Autodesk Inventor part; units mm, degrees
ref_plane "YZ Plane" through (0, 0, 0) normal (1, 0, 0) x (0, 1, 0)
ref_plane "XZ Plane" through (0, 0, 0) normal (0, 1, 0) x (-1, 0, 0)
ref_plane "XY Plane" through (0, 0, 0) normal (0, 0, 1) x (1, 0, 0)
sketch "Sketch1" plane through (0, 0, 0) normal (0, 0, 1) x (1, 0, 0)
  circle A0 centre (0, 0) radius 11
  circle A1 centre (0, 0) radius 18
  circle A2 centre (0, 0) radius 13
  dimension "d0" = 22
  dimension "d2" = 2
  dimension "d3" = 5
extrude "Extrusion1" add sketch "Sketch1" along normal mid plane 10 contours A1 | A2
extrude "Extrusion2" cut sketch "Sketch1" along normal mid plane 7 contours A1
sketch "Sketch2" plane through (0, 0, -5) normal (0, 0, -1) x (-1, 0, 0)
  circle A0 centre (0, 0) radius 4
  circle A1 centre (0, 0) radius 18
  dimension "d8" = 8
extrude "Extrusion3" add sketch "Sketch2" along normal blind 1
properties part number "Belt Tensioner" material "PC/ABS Plastic"
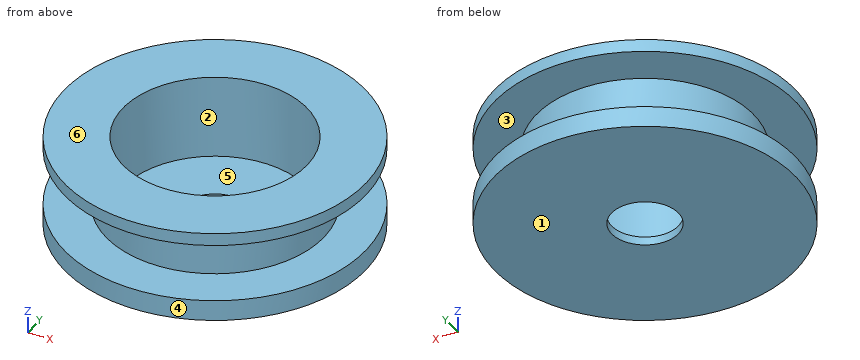
Source: CAD feature listing. Evaluate the final solid. Frame: model axes, mm. Face numbers are marked on the shaded views. A direction names the side the tool comes from. Give positions to 0.01 mm unless a question says otherwise; leave off trailing zeros. Write each loop counter-clockwise with the first axis right and the second up, starting at its lowest first coordinate (ties: lowest second). Pieces come first, ordered by that corner, then holes.
1. Section query D-D (x = 5.5). Return the cut outline in (y, z), then the cut area to 3 significant figures.
2. Pull-direction query (X, two-part tool) for the marked faces 4, 5 and 6; classes: +X half, -X half, draft (parallel to the pull), parting line (faces both ways), or undercut.
3. First-contact query: pin 1 (9 mm diameter, centred on x = 0, y = 0, fed in from +Z); pin 2 (6 mm diameter, centred on y = -6.5, z = 2, fed in from +X); pin 3 (1.5 mm diameter, centred on y = 9, z = 4, fed in from -X). Flat tips, straight axial feed; report the tip coordinate or a pass-through.
4. Section query C-C (z = -0.25). Return the cut outline in (x, y).
5. Access query for the marked faces 1, 2 and 3. Directions: +Z, -Z, +X, -X, +Y, -Y. A direction counts if a zero-diameter tool reaches every point of the face in a straight line with its end or side. Return the directions, or none.
6. Material intervals for line 1 along Y through (x, z) = (0, -5.2); line 2 along Z through (x, y) = (-11, -11); line 3 along Y through (x, z) = (0, 1.25), sorted ascending.
7. Section query A-A (y = 0). Return the cut outline in (x, z).
Output values:
1. outline: (-17.14, -6) - (17.14, -6) - (17.14, -3.5) - (11.78, -3.5) - (11.78, 3.5) - (17.14, 3.5) - (17.14, 5) - (9.53, 5) - (9.53, -5) - (-9.53, -5) - (-9.53, 5) - (-17.14, 5) - (-17.14, 3.5) - (-11.78, 3.5) - (-11.78, -3.5) - (-17.14, -3.5) - close
1. area: 111 mm2
2. face 4: parting line
2. face 5: undercut
2. face 6: draft
3. pin 1: stops at z = -5
3. pin 2: stops at x = 17.57
3. pin 3: stops at x = -16
4. outline: circle Ø26 at (0, 0); hole circle Ø22 at (0, 0)
5. face 1: -Z, +X, -X, +Y, -Y
5. face 2: +Z
5. face 3: none
6. line 1: y = -18 to -4, 4 to 18
6. line 2: z = -6 to -3.5, 3.5 to 5
6. line 3: y = -13 to -11, 11 to 13
7. outline: (-18, -6) - (-4, -6) - (-4, -5) - (-11, -5) - (-11, 5) - (-18, 5) - (-18, 3.5) - (-13, 3.5) - (-13, -3.5) - (-18, -3.5) - close; (4, -6) - (18, -6) - (18, -3.5) - (13, -3.5) - (13, 3.5) - (18, 3.5) - (18, 5) - (11, 5) - (11, -5) - (4, -5) - close
